Could you check a few things on this model? Use its own coordinates, in mm. Round coordinates to 2 decimals unless told otherwise and drop trailing zeros. Write each loop counter-clockwise with the first axis right and the second up, starting at its lowest first coordinate (ties: lowest second). Pieces come first, ordered by that corner, then holes. Notation, with made-up numbers: (7, 12) -> (61, 12) arc R20 cw to (61, 45) -> close; hole circle Ø6 at (-37, -24). An arc over 180 degrees is marked (long way). Answer in a Markdown table with one row per item.
from build123d import *

# Parameters (mm, degrees)
BOSS_EXTRUDE1_DEPTH = 25
SKETCH3_W           = 34
SKETCH3_H           = 10
CUT_EXTRUDE1_DEPTH  = 134.88427839
CUT_EXTRUDE2_DEPTH  = 134.88427839
CUT_EXTRUDE3_DEPTH  = 134.88427839
CUT_EXTRUDE4_DEPTH  = 134.88427839
BOSS_EXTRUDE2_DEPTH = 25
BOSS_EXTRUDE3_DEPTH = 25
LPATTERN1_COUNT     = 30
LPATTERN1_PITCH     = 3
CUT_EXTRUDE5_DEPTH  = 138.359842306
CUT_EXTRUDE6_DEPTH  = 138.359842306
CUT_EXTRUDE7_DEPTH  = 138.359842306
CUT_EXTRUDE8_DEPTH  = 138.359842306


with BuildPart() as part:
    # Sketch2 → Boss-Extrude1 (new body)
    with BuildSketch(Plane.XY):
        with BuildLine():
            Line((-15, 0), (15, 0))
            Line((15, 0), (15, 5))
            Line((15, 5), (8, 5))
            Line((8, 5), (8, 10))
            Line((8, 10), (20, 10))
            Line((20, 10), (20, 130))
            ThreePointArc((20, 130), (-9.083269132, 106.055512755), (-20, 70))
            Line((-20, 70), (-20, 10))
            Line((-20, 10), (-8, 10))
            Line((-8, 10), (-8, 5))
            Line((-8, 5), (-15, 5))
            Line((-15, 5), (-15, 0))
        make_face()
    extrude(amount=BOSS_EXTRUDE1_DEPTH)

    # Sketch3 → Cut-Extrude1 (cut, through all)
    with BuildSketch(Plane.XY.offset(25)):
        with Locations((0, 18)):
            Rectangle(SKETCH3_W, SKETCH3_H)
    extrude(amount=-CUT_EXTRUDE1_DEPTH, mode=Mode.SUBTRACT)

    # Sketch4 → Cut-Extrude2 (cut, through all)
    with BuildSketch(Plane.XY.offset(25)):
        Polygon((-17, 26), (17, 26), (17, 36), (-17, 41.995117344), align=None)
    extrude(amount=-CUT_EXTRUDE2_DEPTH, mode=Mode.SUBTRACT)

    # Sketch5 → Cut-Extrude3 (cut, through all)
    with BuildSketch(Plane.XY.offset(25)):
        Polygon((-17, 45.04139718), (17, 39.046279836), (17, 49.046279836), (-17, 61.421267801), align=None)
    extrude(amount=-CUT_EXTRUDE3_DEPTH, mode=Mode.SUBTRACT)

    # Sketch6 → Cut-Extrude4 (cut, through all)
    with BuildSketch(Plane.XY.offset(25)):
        with BuildLine():
            Line((-17, 64.613801118), (17, 52.238813153))
            Line((17, 52.238813153), (17, 62.238813153))
            Line((17, 62.238813153), (-15.966701553, 81.272147169))
            ThreePointArc((-15.966701553, 81.272147169), (-16.741134976, 75.659704221), (-17, 70))
            Line((-17, 70), (-17, 64.613801118))
        make_face()
    extrude(amount=-CUT_EXTRUDE4_DEPTH, mode=Mode.SUBTRACT)

    # Sketch13 → Boss-Extrude2 (add)
    with BuildSketch(Plane.XY.offset(25)):
        with BuildLine():
            Line((28.543587015, 132.015112463), (28.543587015, 130.015112463))
            ThreePointArc((28.543587015, 130.015112463), (22.183163486, 116.610368534), (20, 101.934676234))
            Line((20, 101.934676234), (20, 130))
            ThreePointArc((20, 130), (24.189413282, 131.356828362), (28.543587015, 132.015112463))
        make_face()
    extrude(amount=-BOSS_EXTRUDE2_DEPTH)

    # Sketch15 → Boss-Extrude3 (add)
    with BuildSketch(Plane.XY.offset(25)):
        Polygon((20, 101.934676234), (22.598076211, 100.434676234), (20, 98.934676234), align=None)
    boss_extrude3 = extrude(amount=-BOSS_EXTRUDE3_DEPTH)

    # LPattern1: Boss-Extrude3 ×30
    with Locations(*[(0, -i * LPATTERN1_PITCH, 0) for i in range(1, LPATTERN1_COUNT)]):
        add(boss_extrude3)

    # Sketch17 → Cut-Extrude5 (cut, through all)
    with BuildSketch(Plane.XY.offset(25)):
        with BuildLine():
            Line((-15.314209237, 84.35953217), (17, 65.702914768))
            Line((17, 65.702914768), (17, 75.702914768))
            Line((17, 75.702914768), (-10.093752299, 98.43727233))
            ThreePointArc((-10.093752299, 98.43727233), (-13.131704676, 91.557015366), (-15.314209237, 84.35953217))
        make_face()
    extrude(amount=-CUT_EXTRUDE5_DEPTH, mode=Mode.SUBTRACT)

    # Sketch18 → Cut-Extrude6 (cut, through all)
    with BuildSketch(Plane.XY.offset(25)):
        with BuildLine():
            Line((-8.623988609, 101.120216028), (17, 79.619136636))
            Line((17, 79.619136636), (17, 89.619136636))
            Line((17, 89.619136636), (-1.21635527, 111.328543473))
            ThreePointArc((-1.21635527, 111.328543473), (-5.18043497, 106.413238612), (-8.623988609, 101.120216028))
        make_face()
    extrude(amount=-CUT_EXTRUDE6_DEPTH, mode=Mode.SUBTRACT)

    # Sketch19 → Cut-Extrude7 (cut, through all)
    with BuildSketch(Plane.XY.offset(25)):
        with BuildLine():
            Line((0.851852517, 113.530920893), (17, 94.286308117))
            Line((17, 94.286308117), (17, 104.286308117))
            Line((17, 104.286308117), (8.050664287, 119.787012266))
            ThreePointArc((8.050664287, 119.787012266), (4.330784185, 116.797594863), (0.851852517, 113.530920893))
        make_face()
    extrude(amount=-CUT_EXTRUDE7_DEPTH, mode=Mode.SUBTRACT)

    # Sketch21 → Cut-Extrude8 (cut, through all)
    with BuildSketch(Plane.XY.offset(25)):
        with BuildLine():
            Line((10.512523927, 121.522946287), (17, 110.286308117))
            Line((17, 110.286308117), (17, 125.317266744))
            ThreePointArc((17, 125.317266744), (13.698715946, 123.518497892), (10.512523927, 121.522946287))
        make_face()
    extrude(amount=-CUT_EXTRUDE8_DEPTH, mode=Mode.SUBTRACT)


solid = part.part
1) For pin 1 (5.5 mm diameter, centred on y = 1.5, z = 14.5, fed in from +X); pin 2 (1 mm diameter, centred on x = 9.5, z = 14, fed in from +Y); pin 3 (5 mm diameter, centred on y = 53, z = 14, fed in from +X), each with a flat end and sliding along its axis, tell me the tip position at first contact or that it passes through.
Findings:
| item | result |
|---|---|
| pin 1 | stops at x = 15 |
| pin 2 | stops at y = 124.77 |
| pin 3 | stops at x = 22.6 |
2) Imagine slicing it at A-A, the plane y = 106. Please give me the cut outline in (x, z).
Findings:
| item | result |
|---|---|
| outline | (-9.12, 0) -> (-5.48, 0) -> (-5.48, 25) -> (-9.12, 25) -> close; (3.25, 0) -> (7.17, 0) -> (7.17, 25) -> (3.25, 25) -> close; (16.01, 0) -> (20.16, 0) -> (20.16, 25) -> (16.01, 25) -> close |
3) Imagine slicing it at B-B, the plane y = 123. Please give me the cut outline in (x, z).
Findings:
| item | result |
|---|---|
| outline | (7.37, 0) -> (12.83, 0) -> (12.83, 25) -> (7.37, 25) -> close; (17, 0) -> (24.61, 0) -> (24.61, 25) -> (17, 25) -> close |
4) Please list where these lines run through material, in increasing order: line 1 (X direction, y = 100.5, z = 3.25); line 2 (X direction, y = 77, z = 16); line 3 (X direction, y = 7.5, z = 23.5).
Findings:
| item | result |
|---|---|
| line 1 | x = -12.4 to -7.88, 7.87 to 11.79, 17 to 22.48 |
| line 2 | x = -19.62 to -16.6, -8.57 to -2.57, 15.45 to 21.62 |
| line 3 | x = -8 to 8 |
5) Imagine slicing it at C-C, the plane z = 1.5. Count the separate pieces of the cut face and the enclosed holes in it, plus the area to 3 significant figures.
Findings:
| item | result |
|---|---|
| separate pieces | 1 |
| enclosed holes | 8 |
| area | 1,940 mm^2 |
6) Thinking about a two-plate mould opening in Y: for faces 1 (the face through (21.317, 12.695, 12.675)), 2 (the face through (3.643, 86.911, 12.675)), 3 (the face through (0.62, 75.16, 12.68)), which applies, +Y half, -Y half, draft (parallel to the pull), parting line (faces both ways), or undercut?
Findings:
| item | result |
|---|---|
| face 1 | -Y half |
| face 2 | undercut |
| face 3 | undercut |
